from build123d import *

# Parameters (mm, degrees)
F_4_0_4_HEAT_INSERT_M3_D         = 4
F_8_1_8_1_DURCHMESSER_BOHRUNG1_D = 8.1
SKIZZE8_R                        = 1.2
SCHNITT_LINEAR_AUSTRAGEN1_DEPTH  = 7
KREISMUSTER1_COUNT               = 5


with BuildPart() as part:
    # Skizze1 → Rotation1 (revolve)
    with BuildSketch(Plane(origin=(0, 0, 0), x_dir=(0, 0, -1), z_dir=(1, 0, 0)), mode=Mode.PRIVATE) as rotation1_sk:
        Polygon((0, 0), (20, 0), (20, 15), (8, 15), (8, 32.5), (0, 32.5), align=None)
    revolve(rotation1_sk.sketch.rotate(Axis((0, 0, 0), (0, 0, 1)), 90), axis=Axis((0, 0, 0), (0, 0, 1)))

    # Ø4.0 (4) Heat Insert M3 (through all)
    with Locations(Plane.XY):
        with Locations((0, 22.5)):
            f_4_0_4_heat_insert_m3 = Hole(F_4_0_4_HEAT_INSERT_M3_D / 2)

    # Ø8.1 (8.1) Durchmesser Bohrung1 (through all)
    with Locations(Plane.XY):
        with Locations((0, 0)):
            Hole(F_8_1_8_1_DURCHMESSER_BOHRUNG1_D / 2)

    # Skizze8 → Schnitt-Linear austragen1 (cut)
    with BuildSketch(Plane(origin=(0, 0, -20), x_dir=(-1, 0, 0), z_dir=(0, 0, -1))):
        with Locations((0, 10)):
            Circle(SKIZZE8_R)
        with Locations((8.660254038, -5)):
            Circle(SKIZZE8_R)
        with Locations((-8.660254038, -5)):
            Circle(SKIZZE8_R)
    extrude(amount=-SCHNITT_LINEAR_AUSTRAGEN1_DEPTH, mode=Mode.SUBTRACT)

    # Kreismuster1: Ø4.0 (4) Heat Insert M3 ×5 about axis
    kreismuster1_axis = Axis((0, 0, 0), (0, 0, 1))
    for i in range(1, KREISMUSTER1_COUNT):
        add(f_4_0_4_heat_insert_m3.rotate(kreismuster1_axis, i * 360 / KREISMUSTER1_COUNT), mode=Mode.SUBTRACT)


solid = part.part
Verification items for the finished model (mm, model axes). A direction names the side the tool comes from. Coordinates: 2 decimals unless noted, no trailing zeros. Write each loop counter-clockwise with the first axis right and the second up, starting at its lowest first coordinate (ties: lowest second). Pieces come first, ordered by that corner, then holes. Notation, with made-up numbers: M -6.5,-25.75 L 51.5,-25.75 A20 ccw 51.5,8.25 Z; hole C 37.5,81 d5. An arc over 180 degrees is marked long. Use a Markdown table: item, result.
Q1. Thickness scan on line 1 (Z direction, x = -11.5, y = 16.5); line 2 (X direction, y = 2, z = -18); line 3 (Y direction, x = 18, z = -3.5). Record the ranges inside material, lowest first.
Reply:
| item | result |
|---|---|
| line 1 | z = -8 to 0 |
| line 2 | x = -14.87 to -3.52, 3.52 to 14.87 |
| line 3 | y = -27.06 to 27.06 |
Q2. Sectioned sample at C-C, the plane y = 6. Record the boundary of the cut face in (x, z), plus the area to 3 significant figures.
Reply:
| item | result |
|---|---|
| outline | M -31.94,-8 L -23.16,-8 L -23.16,0 L -31.94,0 Z; M -19.64,-8 L -13.75,-8 L -13.75,-20 L 13.75,-20 L 13.75,-8 L 19.64,-8 L 19.64,0 L -19.64,0 Z; M 23.16,-8 L 31.94,-8 L 31.94,0 L 23.16,0 Z |
| area | 785 mm² |
Q3. Sectioned sample at B-B, the plane y = 22.5. Record the boundary of the cut face in (x, z), plus the area to 3 significant figures.
Reply:
| item | result |
|---|---|
| outline | M -23.45,-8 L -2,-8 L -2,0 L -23.45,0 Z; M 2,-8 L 23.45,-8 L 23.45,0 L 2,0 Z |
| area | 343 mm² |
Q4. Draft check along Y on faces 3 (the face through (0.878, -3.954, -10.14)), 4 (the face through (-31, -9.76, -3.94)), 5 (the face through (-7, 0, 0)). Enter one of: +Y half, -Y half, draft (parallel to the pull), parting line (faces both ways), or undercut.
Reply:
| item | result |
|---|---|
| face 3 | undercut |
| face 4 | parting line |
| face 5 | draft |
Q5. Set-up check for faces 1 (the face through (-9, -5, -13)), 2 (the face through (19.426, 7.282, -4.056)): record each of +Z, -Z, +X, -X, +Y, -Y from which the full face is reachable in a straight line by a thin tool's end or side.
Reply:
| item | result |
|---|---|
| face 1 | -Z |
| face 2 | +Z, -Z |
Q6. Sectioned sample at A-A, the plane x = 0. Record the boundary of the cut face in (y, z).
Reply:
| item | result |
|---|---|
| outline | M -32.5,-8 L -15,-8 L -15,-20 L -4.05,-20 L -4.05,0 L -32.5,0 Z; M 4.05,-20 L 8.8,-20 L 8.8,-13 L 11.2,-13 L 11.2,-20 L 15,-20 L 15,-8 L 20.5,-8 L 20.5,0 L 4.05,0 Z; M 24.5,-8 L 32.5,-8 L 32.5,0 L 24.5,0 Z |
Q7. Go/stop test with flat-tipped pins: P1, Ø5, axis at y = -8.5, z = -15.5, coming from the -X side; P2, Ø3, axis at y = -12.5, z = -12, coming from the -X side; P3, Ø4.5, axis at x = -21.4, y = 6.95, coming from the -Z side. Record where each tip stops, or that it passes through.
Reply:
| item | result |
|---|---|
| P1 | stops at x = -13.75 |
| P2 | stops at x = -10.2 |
| P3 | stops at z = -8 |
Q8. Sectioned sample at D-D, the plane z = -15.5. Record the boundary of the cut face in (x, y), plus the area to 3 significant figures.
Reply:
| item | result |
|---|---|
| outline | C 0,0 d30; hole C -8.66,-5 d2.4; hole C 0,0 d8.1; hole C 0,10 d2.4; hole C 8.66,-5 d2.4 |
| area | 642 mm² |
